from build123d import *

# Parameters (mm, degrees)
SKETCH1_W                                       = 317.5
SKETCH1_H                                       = 50.8
BOSS_EXTRUDE1_DEPTH                             = 6.35
CBORE_FOR_10_SOCKET_HEAD_CAP_SCREW1_D           = 5.1054
CBORE_FOR_10_SOCKET_HEAD_CAP_SCREW1_CBORE_D     = 9.525
CBORE_FOR_10_SOCKET_HEAD_CAP_SCREW1_CBORE_DEPTH = 2.54
F_1_4_CLEARANCE_HOLE2_D                         = 6.7564
F_6_32_TAPPED_HOLE1_D                           = 2.7051
SKETCH12_W                                      = 25.4
SKETCH12_H                                      = 25.4
BOSS_EXTRUDE3_DEPTH                             = 6.35
F_10_32_TAPPED_HOLE1_D                          = 4.0386
FILLET1_R                                       = 12.7
FILLET2_R                                       = 2.54


with BuildPart() as part:
    # Sketch1 → Boss-Extrude1 (new body)
    with BuildSketch(Plane(origin=(0, 0, 0), x_dir=(1, 0, 0), z_dir=(0, 1, 0))):
        Rectangle(SKETCH1_W, SKETCH1_H)
    extrude(amount=BOSS_EXTRUDE1_DEPTH)

    # CBORE for #10 Socket Head Cap Screw1 (through all)
    with Locations(Plane(origin=(0, 6.35, 0), x_dir=(1, 0, 0), z_dir=(0, 1, 0))):
        with Locations((31.75, -12.7), (19.05, 12.7), (69.85, 12.7), (19.05, -12.7), (69.85, -12.7), (-125.73, 12.7), (-125.73, 0), (-125.73, -12.7), (31.75, 12.7)):
            CounterBoreHole(CBORE_FOR_10_SOCKET_HEAD_CAP_SCREW1_D / 2, CBORE_FOR_10_SOCKET_HEAD_CAP_SCREW1_CBORE_D / 2, CBORE_FOR_10_SOCKET_HEAD_CAP_SCREW1_CBORE_DEPTH)

    # 1/4 Clearance Hole2 (through all)
    with Locations(Plane.XZ):
        with Locations((-146.05, 12.7), (-146.05, 0), (-146.05, -12.7), (149.225, 12.7), (149.225, 0), (149.225, -12.7)):
            Hole(F_1_4_CLEARANCE_HOLE2_D / 2)

    # #6-32 Tapped Hole1 (through all)
    with Locations(Plane(origin=(0, 0, 0), x_dir=(-1, 0, 0), z_dir=(0, -1, 0))):
        with Locations((57.15, 0)):
            Hole(F_6_32_TAPPED_HOLE1_D / 2)

    # Sketch12 → Boss-Extrude3 (add)
    with BuildSketch(Plane(origin=(0, 6.35, 0), x_dir=(1, 0, 0), z_dir=(0, 1, 0))):
        with Locations((-57.15, 38.1)):
            Rectangle(SKETCH12_W, SKETCH12_H)
    extrude(amount=-BOSS_EXTRUDE3_DEPTH)

    # #10-32 Tapped Hole1 (through all)
    with Locations(Plane(origin=(0, 0, 0), x_dir=(-1, 0, 0), z_dir=(0, -1, 0))):
        with Locations((59.055, 43.18), (55.245, 33.02)):
            Hole(F_10_32_TAPPED_HOLE1_D / 2)

    # Fillet1
    fillet1_edges = [part.edges().sort_by_distance(p)[0] for p in [
        (-69.85, 3.175, -25.4),
        (-44.45, 3.175, -25.4),
    ]]
    fillet(fillet1_edges, radius=FILLET1_R)

    # Fillet2
    fillet2_edges = [part.edges().sort_by_distance(p)[0] for p in [
        (-44.45, 3.175, -50.8),
        (-69.85, 3.175, -50.8),
        (158.75, 3.175, 25.4),
        (-158.75, 3.175, 25.4),
        (-158.75, 3.175, -25.4),
        (158.75, 3.175, -25.4),
    ]]
    fillet(fillet2_edges, radius=FILLET2_R)


solid = part.part
Verification items for the finished model (mm, model axes). A direction names the side the tool comes from. Round coordinates to 2 decimals unless told otherwise and drop trailing zeros. Order: outer loops, then holes, each group sorted by start corner. A loop starts at its lowest first (then second) coordinate and runs counter-clockwise, first axis right, second up. Notation, with made-up numbers: (-23.75, 67.25) -> (-7.75, 67.25) arc R10 ccw to (-7.75, 72.25) -> close; hole circle Ø6 at (-19.5, 86). An arc over 180 degrees is marked (long way). Put each result on its own line as item: value.
1) Section check A-A (y = 1.5). Give the number of separate pieces and of enclosed holes in the cut face, then the cut area to 3 significant figures.
Final values:
separate pieces: 1
enclosed holes: 18
area: 16,400 mm^2
2) Section check C-C (x = 95.5). Record the cut outline in (y, z).
Final values:
outline: (0, -25.4) -> (6.35, -25.4) -> (6.35, 25.4) -> (0, 25.4) -> close
3) Section check B-B (x = -146.05). Record the cut outline in (y, z), then the cut area to 3 significant figures.
Final values:
outline: (0, -25.4) -> (6.35, -25.4) -> (6.35, -16.08) -> (0, -16.08) -> close; (0, -9.32) -> (6.35, -9.32) -> (6.35, -3.38) -> (0, -3.38) -> close; (0, 3.38) -> (6.35, 3.38) -> (6.35, 9.32) -> (0, 9.32) -> close; (0, 16.08) -> (6.35, 16.08) -> (6.35, 25.4) -> (0, 25.4) -> close
area: 194 mm^2
4) Depth check by flat-ended pin: pin 1 (4 mm diameter, centred on x = 149.225, z = 0, fed in from -Y); pin 2 (8.5 mm diameter, centred on x = -125.73, z = 12.7, fed in from -Y); pin 3 (5 mm diameter, centred on x = 18.5, z = -13.5, fed in from +Y). Enter the tip coordinate at first touch or a pass-through.
Final values:
pin 1: passes through
pin 2: stops at y = 0
pin 3: stops at y = 3.81
5) Mould release check, pull along Z, two halves, no side actions. Record for faces 1 (the flat face through (-69.85, 3, -43)), 2 (the cylindrical face through (36.3, 5.1, 11.3)), 3 (the cylindrical face through (-40.63, 3.13, -29.02)): +Z half, -Z half, draft (parallel to the pull), parting line (faces both ways), or undercut.
Final values:
face 1: draft
face 2: undercut
face 3: -Z half
6) Material ranges on line 1 (Z direction, x = 19.5, y = 3.75); line 2 (Z direction, x = -125.73, y = 2.2); line 3 (Z direction, x = 69.85, y = 4.3), recorded low to high.
Final values:
line 1: z = -25.4 to -15.21, -10.19 to 10.19, 15.21 to 25.4
line 2: z = -25.4 to -15.25, -10.15 to -2.55, 2.55 to 10.15, 15.25 to 25.4
line 3: z = -25.4 to -17.46, -7.94 to 7.94, 17.46 to 25.4
7) Set-up check for faces 4 (the cylindrical face through (29.4, 1.9, -11.7)), 5 (the flat face through (-120, 3, -25.4)), 6 (the flat face through (-123.7, 3.81, 2)): record each of +Z, -Z, +X, -X, +Y, -Y from which the full face is reachable in a straight line by a thin tool's end or side.
Final values:
face 4: +Y, -Y
face 5: -Z, -X, +Y, -Y
face 6: +Y
